Read the model definition and answer for the solid it produces. Units are mm, in the model's axes. Face numbers are marked on the shaded views. Coordinates: 2 decimals unless noted, no trailing zeros. Loops run counter-clockwise (first coordinate to the right, second up) from the corner with the lowest first, then second, coordinate; pieces in that order, holes last. Notation, with made-up numbers: (35, 75) -> (88, 75) arc R15 cw to (88, 99) -> close; hole circle Ø2 at (-18, 9). An arc over 180 degrees is marked (long way). Answer as a JSON object with one key per item and string values. Group by question number.
Q1. Determine the mould class of the marked faces 1, 2, 3 and 4 for opening direction Z: released by +Z, released by -Z, zero draft, split by the parting line, or undercut.
Q2. The part is cut by section C-C on y = -3.75. Write down the section's boundary in (x, z), and give its area (3 significant figures).
Q3. The part is cut by section B-B on z = 0. Write down the section's boundary in (x, y).
Q4. Straight lines are drawn through the part: line 1 along X through (y, z) = (-0.65, -1); line 2 along X through (y, z) = (-4.3, 0.5); line 3 along Y through (x, z) = (20.25, -2.25). For each, find the intervals that lie inside material, in ascending order. Write a range as [from, to].
Q5. The part is cut by section D-D on x = 0. Write down the section's boundary in (y, z).
Q6. The part is cut by section A-A on x = 18.5. Write down the section's boundary in (y, z).
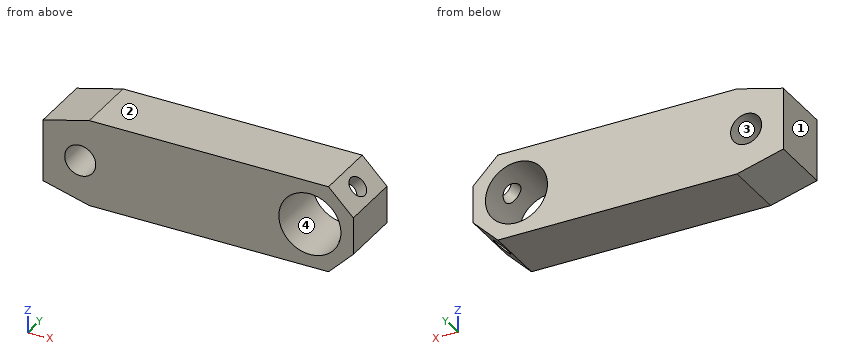
from build123d import *

# Parameters (mm, degrees)
BLOCK_R                = 2.5
BOSS_EXTRUDE1_DEPTH    = 5
M3_TAPPED_HOLE1_D      = 2.5
M2_TAPPED_HOLE1_REACH  = 23.797
M2_TAPPED_HOLE1_BORE_R = 0.8


with BuildPart() as part:
    # block → Boss-Extrude1 (new body)
    with BuildSketch(Plane(origin=(0, 0, 0), x_dir=(1, 0, 0), z_dir=(0, 1, 0))):
        Polygon((0.732050808, 3.5), (20, 3.5), (22, 1.5), (22, -1.5), (20, -3.5), (0.732050808, -3.5), (-3, -2.5), (-3, 2.5), align=None)
        with Locations(Location((18.5, 0, 0), (0, 0, 270))):
            Circle(BLOCK_R, mode=Mode.SUBTRACT)
    extrude(amount=-BOSS_EXTRUDE1_DEPTH)

    # M3 Tapped Hole1 (through all)
    with Locations(Plane(origin=(0, 0, 0), x_dir=(1, 0, 0), z_dir=(0, 1, 0))):
        with Locations((0, 0)):
            Hole(M3_TAPPED_HOLE1_D / 2)

    # M2 Tapped Hole1 bore → M2 Tapped Hole1 (cut, up to next)
    with BuildSketch(Plane(origin=(11.75, 0, -11.75), x_dir=(-0.7071067811865465, 0, -0.7071067811865486), z_dir=(0.7071067811865486, 0, -0.7071067811865465)), mode=Mode.PRIVATE) as m2_tapped_hole1_sk1:
        with Locations((-13.081475452, -2.5)):
            Circle(M2_TAPPED_HOLE1_BORE_R)
    m2_tapped_hole1_tool1 = extrude(m2_tapped_hole1_sk1.sketch, amount=-M2_TAPPED_HOLE1_REACH, mode=Mode.PRIVATE) & part.part
    m2_tapped_hole1 = m2_tapped_hole1_tool1.solids().sort_by_distance((21, -2.5, -2.5))[0]
    add(m2_tapped_hole1, mode=Mode.SUBTRACT)

    # Mirror1: M2 Tapped Hole1 across plane
    add(m2_tapped_hole1.mirror(Plane.XY), mode=Mode.SUBTRACT)


solid = part.part
Final values:
{
 "1": {"face 1": "zero draft", "face 2": "released by +Z", "face 3": "undercut", "face 4": "undercut"},
 "2": {"outline": "(-3, -2.5) -> (0.73, -3.5) -> (20, -3.5) -> (22, -1.5) -> (22, 1.5) -> (20, 3.5) -> (0.73, 3.5) -> (-3, 2.5) -> close; hole circle Ø2.5 at (0, 0); hole circle Ø5 at (18.5, 0)", "area": "143 mm2"},
 "3": {"outline": "(-3, -5) -> (-1.25, -5) -> (-1.25, 0) -> (-3, 0) -> close; (1.25, -5) -> (16, -5) -> (16, 0) -> (1.25, 0) -> close; (21, -5) -> (22, -5) -> (22, 0) -> (21, 0) -> close"},
 "4": {"line 1": "x = [-3, -0.75], [0.75, 16.21], [20.79, 22]", "line 2": "x = [-3, -1.15], [1.15, 16.05], [20.95, 22]", "line 3": "y = [-5, -3.22], [-1.78, 0]"},
 "5": {"outline": "(-5, -3.3) -> (0, -3.3) -> (0, -1.25) -> (-5, -1.25) -> close; (-5, 1.25) -> (0, 1.25) -> (0, 3.3) -> (-5, 3.3) -> close"},
 "6": {"outline": "(-5, -3.5) -> (0, -3.5) -> (0, -2.5) -> (-5, -2.5) -> close; (-5, 2.5) -> (0, 2.5) -> (0, 3.5) -> (-5, 3.5) -> close"}
}
